Read the model definition and answer for the solid it produces. Units are mm, in the model's axes. A direction names the side the tool comes from. Round coordinates to 2 decimals unless told otherwise and drop trailing zeros. Write each loop counter-clockwise with the first axis right and the second up, starting at its lowest first coordinate (ties: lowest second). Pieces come first, ordered by that corner, then holes. Notation, with made-up numbers: (-23.5, 26.5) -> (33.5, 26.5) arc R21 ccw to (33.5, 32.5) -> close; hole circle Ø7 at (37.25, 26.25). An arc over 180 degrees is marked (long way). Return JSON: item names as keys, results as strings.
from build123d import *

# Parameters (mm, degrees)
SKETCH1_W               = 25.4
SKETCH1_H               = 25.4
SKETCH1_W_2             = 23.4
SKETCH1_H_2             = 23.4
BOSS_EXTRUDE1_DEPTH     = 110.8
CUT_EXTRUDE1_DEPTH      = 115.38133589
CUT_EXTRUDE1_DEPTH_BACK = 115.38133589
SKETCH2_R               = 2


with BuildPart() as part:
    # Sketch1 → Boss-Extrude1 (new body)
    with BuildSketch(Plane(origin=(0, 0, 0), x_dir=(0, 0, -1), z_dir=(1, 0, 0))):
        Rectangle(SKETCH1_W, SKETCH1_H)
        Rectangle(SKETCH1_W_2, SKETCH1_H_2, mode=Mode.SUBTRACT)
    extrude(amount=BOSS_EXTRUDE1_DEPTH)

    # Sketch2 → Cut-Extrude1 (cut, two sides: drawn at the far end of the back side and taken through both)
    with BuildSketch(Plane.XY.offset(12.7).offset(-CUT_EXTRUDE1_DEPTH_BACK)):
        with Locations(Location((92.1, 0, 0), (0, 0, 180))):
            Circle(SKETCH2_R)
        with Locations(Location((104.1, 0, 0), (0, 0, 180))):
            Circle(SKETCH2_R)
        with Locations(Location((6.7, 0, 0), (0, 0, 180))):
            Circle(SKETCH2_R)
        with Locations(Location((18.7, 0, 0), (0, 0, 180))):
            Circle(SKETCH2_R)
    extrude(amount=CUT_EXTRUDE1_DEPTH + CUT_EXTRUDE1_DEPTH_BACK, mode=Mode.SUBTRACT)


solid = part.part
Item 1: For a pull along X with two mould halves and no side action, classify faces 3 (the flat face through (55, -11.7, 0)), 4 (the flat face through (0, -12, 1)), 5 (the cylindrical face through (94.098, -0.088, 12.193)) as released by +X, released by -X, zero draft, split by the parting line, or undercut.
Worked answers:
{"face 3": "zero draft", "face 4": "released by -X", "face 5": "undercut"}
Item 2: A flat-ended cylindrical pin translates along its axis: pin 1 (3.5 mm diameter, centred on x = 6.7, y = 0, fed in from -Z). Find the tip coordinate at first contact, or state that the pin passes through.
Worked answers:
{"pin 1": "passes through"}
Item 3: Section D-D (x = 86) is taken. Give the vertices of the cut face in (y, z).
Worked answers:
{"outline": "(-12.7, -12.7) -> (12.7, -12.7) -> (12.7, 12.7) -> (-12.7, 12.7) -> close; hole (-11.7, -11.7) -> (11.7, -11.7) -> (11.7, 11.7) -> (-11.7, 11.7) -> close"}
Item 4: Straight lines are drawn through the part: L1, parallel to Y at x = 75, z = 6; L2, parallel to Y at x = 6.7, z = -11.9. For each, find the intervals that lie inside material, in ascending order. Write a range as [from, to].
Worked answers:
{"L1": "y = [-12.7, -11.7], [11.7, 12.7]", "L2": "y = [-12.7, -2], [2, 12.7]"}
Item 5: A tool of negligible diameter and unlimited length cuts with its end or side. For faces 1 (the flat face through (55, 0, 11.7)), 2 (the cylindrical face through (20.698, -0.088, 12.193)), from which of +Z, -Z, +X, -X, +Y, -Y can it reach the whole face along a straight path? Write none if from no direction.
Worked answers:
{"face 1": "+X, -X", "face 2": "+Z, -Z"}
Item 6: Section A-A (y = 7.75) is taken. Give the vertices of the cut face in (x, z), then the cut area to 3 significant figures.
Worked answers:
{"outline": "(0, -12.7) -> (110.8, -12.7) -> (110.8, -11.7) -> (0, -11.7) -> close; (0, 11.7) -> (110.8, 11.7) -> (110.8, 12.7) -> (0, 12.7) -> close", "area": "222 mm2"}
Item 7: Section B-B (x = 18.7) is taken. Give the vertices of the cut face in (y, z).
Worked answers:
{"outline": "(-12.7, -12.7) -> (-2, -12.7) -> (-2, -11.7) -> (-11.7, -11.7) -> (-11.7, 11.7) -> (-2, 11.7) -> (-2, 12.7) -> (-12.7, 12.7) -> close; (2, -12.7) -> (12.7, -12.7) -> (12.7, 12.7) -> (2, 12.7) -> (2, 11.7) -> (11.7, 11.7) -> (11.7, -11.7) -> (2, -11.7) -> close"}
